Check sheet for the modelled part. Datum: model origin and axes. Units: mm. A direction names the side the tool comes from. Round coordinates to 2 decimals unless told otherwise and drop trailing zeros. Order: outer loops, then holes, each group sorted by start corner. A loop starts at its lowest first (then second) coordinate and runs counter-clockwise, first axis right, second up. Notation, with made-up numbers: (2, 43) -> (50, 43) arc R13 ccw to (50, 61) -> close; hole circle Ø2 at (23.25, 86.5). An arc over 180 degrees is marked (long way). Answer in a Markdown table with one row per item.
Autodesk Inventor part; units mm, degrees
ref_plane "bolt_to_nut_XY" through (45, 0, 0) normal (1, 0, 0) x (0, 0, -1)
ref_plane "bolt_to_nut_YZ" through (45, 0, 0) normal (0, 0, -1) x (0, 1, 0)
ref_plane "bolt_to_nut_ZX" through (45, 0, 0) normal (0, 1, 0) x (1, 0, 0)
sketch "Sketch_2" plane through (0, 0, 0) normal (0, 0, 1) x (1, 0, 0)
  line L0 (45, 0) -> (-4, 0)
  line L1 (-4, 0) -> (-4, 3.1)
  line L2 (-4, 3.1) -> (-3.6, 3.5)
  line L3 (-3.6, 3.5) -> (0, 3.5)
  line L4 (0, 3.5) -> (0, 2)
  line L5 (0, 2) -> (44.5705, 2)
  line L6 (44.5705, 2) -> (45, 1.5705)
  line L7 (45, 1.5705) -> (45, 0)
  line L8 (45, 0) -> (-4, 0)
revolve "Revolution1" add sketch "Sketch_2" angle 360 about axis through (45, 0, 0) along (1, 0, 0)
thread "Thread1"
sketch "Sketch2" plane through (-4, 0, 0) normal (-1, 0, 0) x (0, 0, 1)
  point P0 (0, 0)
hole "Hole1" at (-4, 0, 0) direction (1, 0, 0) diameter 3 depth 2 tip angle 150
sketch "Sketch_3" plane through (-4, 0, 0) normal (1, 0, 0) x (0, 0, -1)
  line L0 (-1.5, -0.866) -> (0, -1.7321)
  line L1 (0, -1.7321) -> (1.5, -0.866)
  line L2 (1.5, -0.866) -> (1.5, 0.866)
  line L3 (1.5, 0.866) -> (0, 1.7321)
  line L4 (0, 1.7321) -> (-1.5, 0.866)
  line L5 (-1.5, 0.866) -> (-1.5, -0.866)
extrude "Extrusion1" cut sketch "Sketch_3" along normal blind 2
ref_plane "bolt_to_nut_XY" through (45, 0, 0) normal (1, 0, 0) x (0, 0, -1)
ref_plane "bolt_to_nut_YZ" through (45, 0, 0) normal (0, 0, -1) x (0, 1, 0)
ref_plane "bolt_to_nut_ZX" through (45, 0, 0) normal (0, 1, 0) x (1, 0, 0)
ref_plane "screw1_XY" through (0, 0, 0) normal (1, 0, 0) x (0, 0, -1)
ref_plane "screw1_YZ" through (0, 0, 0) normal (0, 0, -1) x (0, 1, 0)
ref_plane "screw1_ZX" through (0, 0, 0) normal (0, 1, 0) x (1, 0, 0)
properties part number "CB4-45" material "鋼、炭素鋼"
(1) Section check A-A on x = 10. Record the boundary of the cut face in (y, z), plus the area to 3 significant figures.
Solutions:
| item | result |
|---|---|
| outline | circle Ø4 at (0, 0) |
| area | 12.6 mm^2 |
(2) Draft check along Y on faces 4 (the flat face through (-3.014, 1.293, -0.76)), 5 (the flat face through (45, 0, 0)), 6 (the cylindrical face through (23, 0, -2)). Enter one of: pulls with the +Y half, pulls with the -Y half, needs draft (parallel to the pull), parting line crosses it, or undercut.
Solutions:
| item | result |
|---|---|
| face 4 | undercut |
| face 5 | needs draft |
| face 6 | parting line crosses it |
(3) Depth check by flat-ended pin: pin 1 Ø2 at (y, z) = (-2, -2) entering from +X; pin 2 Ø0.5 at (y, z) = (0.5, -0.5) entering from -X; pin 3 Ø2 at (x, y) = (17, -2) entering from -Z. Enter the tip coordinate at first touch or a pass-through.
Solutions:
| item | result |
|---|---|
| pin 1 | x = 44.74 |
| pin 2 | x = -1.85 |
| pin 3 | z = -1.73 |
(4) Scan lines: probe 1 along Z at (x, y) = (5.5, 0); probe 2 along X at (y, z) = (0.75, -2.5); probe 3 along Y at (x, z) = (7.5, 1.25). Record each from-to range of solid material in increasing order. Write a range as from..to.
Solutions:
| item | result |
|---|---|
| probe 1 | -2..2 |
| probe 2 | -4..0 |
| probe 3 | -1.56..1.56 |
(5) Tool access check on faces 1 (the flat face through (-3, 0, 1.5)), 2 (the flat face through (0, 2, -2)), 3 (the flat face through (-4, 1.3, -1.3)). Record the directions out of +Z, -Z, +X, -X, +Y, -Y that give a thin tool (end or side, any length) a straight path to the whole face; none if there is none.
Solutions:
| item | result |
|---|---|
| face 1 | -X |
| face 2 | +X |
| face 3 | +Z, -Z, -X, +Y, -Y |
